Could you check a few things on this model? Use its own coordinates, in mm. A direction names the side the tool comes from. Give positions to 0.01 mm unless a question says otherwise; leave off trailing zeros. Order: outer loops, then holes, each group sorted by start corner. A loop starts at its lowest first (then second) coordinate and runs counter-clockwise, first axis right, second up.
(1) Imagine slicing it at D-D, the plane z = 0. Write out the boundary of the cut face in (x, y) (3 decimals).
(2) Imagine slicing it at C-C, the plane x = -30. Write out the boundary of the cut face in (y, z).
(3) If we mould it in two halves opening along Z, with no side actions, what happens to faces 1 (the cylindrical face through (-34.88, 13.97, -1.08)), 2 (the flat face through (5, 0, 0)), 3 (the cylindrical face through (-3.905, 7.28, -0.867))? For each: released by +Z, released by -Z, zero draft, split by the parting line, or undercut.
(4) If I drill on probe 1 along X at (y, z) = (7.75, 0); probe 2 along X at (y, z) = (12.25, 0); probe 3 along Z at (x, y) = (-16, 3.5), over which ranges is the centre line in solid material (lowest first)?
(5) Imagine slicing it at A-A, the plane y = 2.25. Write out the boundary of the cut face in (x, z), then the cut area to 3 significant figures.
(6) Will these pins go through, and if not, where does the flat tip stop? pin 1 (2.5 mm diameter, centred on x = 23.5, y = 2, fed in from +Z); pin 2 (1.5 mm diameter, centred on y = 3, z = 33, fed in from +X); pin 3 (1.5 mm diameter, centred on y = 2.5, z = 42.5, fed in from -X); pin 4 (10 mm diameter, centred on x = -12.5, z = 8.5, fed in from -Y).
(7) On a 3-axis mill with a long thin cutter (end or side, diameter ignored), from which of +Z, -Z, +X, -X, +Y, -Y can I reach the whole of each face in a straight line? I mean faces 4 (the flat face through (0, 10, 0)), 5 (the flat face through (6, 2, 33)), 6 (the cylindrical face through (0, 14, -65)). Say none if no direction works.
(8) Imagine slicing it at B-B, the plane z = -44.5. Write out the boundary of the cut face in (x, y).
from build123d import *

# Parameters (mm, degrees)
SKETCH1_R           = 66
BOSS_EXTRUDE1_DEPTH = 5
FILLET1_R           = 5
SKETCH2_R           = 4
SKETCH2_R_2         = 3
BOSS_EXTRUDE2_DEPTH = 5
CHAMFER1_SIZE       = 0.375
SKETCH3_R           = 5
BOSS_EXTRUDE3_DEPTH = 18.2
SKETCH4_R           = 5
BOSS_EXTRUDE4_DEPTH = 18.2


with BuildPart() as part:
    # Sketch1 → Boss-Extrude1 (new body)
    with BuildSketch(Plane(origin=(0, 0, 0), x_dir=(1, 0, 0), z_dir=(0, 1, 0))):
        with Locations(Location((0, 0, 0), (0, 0, 270))):
            Circle(SKETCH1_R)
        with BuildLine():
            Line((-6, -59.699246226), (-6, -6))
            Line((-6, -6), (-59.699246226, -6))
            ThreePointArc((-59.699246226, -6), (-42.426406871, -42.426406871), (-6, -59.699246226))
        make_face(mode=Mode.SUBTRACT)
        with BuildLine():
            Line((6, -59.699246226), (6, -6))
            Line((6, -6), (59.699246226, -6))
            ThreePointArc((59.699246226, -6), (42.426406871, -42.426406871), (6, -59.699246226))
        make_face(mode=Mode.SUBTRACT)
        with BuildLine():
            Line((-59.699246226, 6), (-6, 6))
            Line((-6, 6), (-6, 59.699246226))
            ThreePointArc((-6, 59.699246226), (-42.426406871, 42.426406871), (-59.699246226, 6))
        make_face(mode=Mode.SUBTRACT)
        with BuildLine():
            Line((6, 6), (6, 59.699246226))
            ThreePointArc((6, 59.699246226), (42.426406871, 42.426406871), (59.699246226, 6))
            Line((59.699246226, 6), (6, 6))
        make_face(mode=Mode.SUBTRACT)
    extrude(amount=BOSS_EXTRUDE1_DEPTH)

    # Fillet1
    fillet1_edges = [part.edges().sort_by_distance(p)[0] for p in [
        (-6, 2.5, -59.699246226),
        (-59.699246226, 2.5, -6),
        (-6, 2.5, -6),
        (6, 2.5, 59.699246226),
        (59.699246226, 2.5, 6),
        (6, 2.5, 6),
        (59.699246226, 2.5, -6),
        (6, 2.5, -59.699246226),
        (6, 2.5, -6),
        (-59.699246226, 2.5, 6),
        (-6, 2.5, 59.699246226),
        (-6, 2.5, 6),
    ]]
    fillet(fillet1_edges, radius=FILLET1_R)

    # Sketch2 → Boss-Extrude2 (add)
    with BuildSketch(Plane(origin=(0, 5, 0), x_dir=(1, 0, 0), z_dir=(0, 1, 0))):
        with Locations(Location((0, 0, 0), (0, 0, 270))):
            Circle(SKETCH2_R)
        with Locations(Location((0, 31.6, 0), (0, 0, 270))):
            Circle(SKETCH2_R_2)
    extrude(amount=BOSS_EXTRUDE2_DEPTH)

    # Chamfer1
    chamfer1_edges = [part.edges().sort_by_distance(p)[0] for p in [
        (0, 10, -4),
        (0, 10, -34.6),
    ]]
    chamfer(chamfer1_edges, length=CHAMFER1_SIZE)

    # Sketch3 → Boss-Extrude3 (add)
    with BuildSketch(Plane(origin=(0, 5, 0), x_dir=(1, 0, 0), z_dir=(0, 1, 0))):
        with Locations(Location((-30, 0, 0), (0, 0, 270))):
            Circle(SKETCH3_R)
    boss_extrude3 = extrude(amount=BOSS_EXTRUDE3_DEPTH)

    # Mirror1: Boss-Extrude3 across plane
    add(boss_extrude3.mirror(Plane(origin=(0, 0, 0), x_dir=(0, 0, 1), z_dir=(1, 0, 0))))

    # Sketch4 → Boss-Extrude4 (add)
    with BuildSketch(Plane(origin=(0, 5, 0), x_dir=(1, 0, 0), z_dir=(0, 1, 0))):
        with Locations(Location((0, 60, 0), (0, 0, 270))):
            Circle(SKETCH4_R)
    extrude(amount=BOSS_EXTRUDE4_DEPTH)


solid = part.part
Answer block:
1. outline: (-66, 0) - (66, 0) - (66, 5) - (35, 5) - (35, 23.2) - (25, 23.2) - (25, 5) - (4, 5) - (4, 9.625) - (3.625, 10) - (-3.625, 10) - (-4, 9.625) - (-4, 5) - (-25, 5) - (-25, 23.2) - (-35, 23.2) - (-35, 5) - (-66, 5) - close
2. outline: (0, -58.79) - (5, -58.79) - (5, -51.96) - (0, -51.96) - close; (0, -6) - (5, -6) - (5, -5) - (23.2, -5) - (23.2, 5) - (5, 5) - (5, 6) - (0, 6) - close; (0, 51.96) - (5, 51.96) - (5, 58.79) - (0, 58.79) - close
3. face 1: split by the parting line
3. face 2: zero draft
3. face 3: undercut
4. probe 1: x = -35 to -25, -4 to 4, 25 to 35
4. probe 2: x = -35 to -25, 25 to 35
4. probe 3: z = -64.03 to -57.83, -6 to 6, 57.83 to 64.03
5. outline: circle Ø132 at (0, 0); hole (-58.79, -12) arc R60 ccw to (-12, -58.79) arc R5 ccw to (-6, -53.89) - (-6, -11) arc R5 ccw to (-11, -6) - (-53.89, -6) arc R5 ccw to start; hole (-58.79, 12) arc R5 ccw to (-53.89, 6) - (-11, 6) arc R5 ccw to (-6, 11) - (-6, 53.89) arc R5 ccw to (-12, 58.79) arc R60 ccw to start; hole (6, -53.89) arc R5 ccw to (12, -58.79) arc R60 ccw to (58.79, -12) arc R5 ccw to (53.89, -6) - (11, -6) arc R5 ccw to (6, -11) - close; hole (6, 11) arc R5 ccw to (11, 6) - (53.89, 6) arc R5 ccw to (58.79, 12) arc R60 ccw to (12, 58.79) arc R5 ccw to (6, 53.89) - close
5. area: 5,190 mm2
6. pin 1: stops at z = 62.14
6. pin 2: stops at x = 57.58
6. pin 3: stops at x = -51.12
6. pin 4: stops at y = 0
7. face 4: +Z, +Y
7. face 5: +Y, -Y
7. face 6: +Y
8. outline: (-48.74, 0) - (-40.25, 0) - (-40.25, 5) - (-48.74, 5) - close; (-6, 0) - (6, 0) - (6, 5) - (-6, 5) - close; (40.25, 0) - (48.74, 0) - (48.74, 5) - (40.25, 5) - close
